Model file for the job. Use its own axes, mm. Round coordinates to 2 decimals unless told otherwise and drop trailing zeros. Loops run counter-clockwise (first coordinate to the right, second up) from the corner with the lowest first, then second, coordinate; pieces in that order, holes last. Notation, with made-up numbers: M 41,30 L 77,30 A23 ccw 77,40 Z; hole C 65,46 d11. An arc over 180 degrees is marked long. Use a Markdown table: item, result. Add a question column.
Q1. Cut at D-D (x = 8). Give the cut face in (y, z), plus the area to 3 significant figures.
Q2. Cut at C-C (x = 18.5). Give the cut face in (y, z).
Q3. Cut at A-A (y = 0). Give the cut face in (x, z).
Q4. Pin check, flat tips, straight feed: pin 1 (10 mm diameter, centred on x = 13.5, z = -24, fed in from -Y); pin 2 (1.5 mm diameter, centred on x = 6.5, y = 10, fed in from -Z); pin 3 (8 mm diameter, centred on x = 15.5, z = 1, fed in from +Y). Stop position of each tip, or through.
Q5. Probe line 1 (Y direction, x = 20.05, z = 0); line 2 (Z direction, x = 3.5, y = -6); line 3 (Y direction, x = 16, z = 4.5). List the from-to ranges inside material, lowest first. Write a range as from..to.
Q6. Mould opens along Z. For faces 1 (the face through (16.626, 21.031, -27.428)), 2 (the face through (11.02, -1.76, -39.96)), 3 (the face through (1, -35, -15)) say: +Z half, -Z half, draft (parallel to the pull), parting line (faces both ways), or undercut.
from build123d import *

# Parameters (mm, degrees)
FILLET1_R = 1.5
FILLET2_R = 0.8
FILLET3_R = 0.4


with BuildPart() as part:
    # Sketch1 → Revolve1 (revolve)
    with BuildSketch(Plane.XY, mode=Mode.PRIVATE) as revolve1_sk:
        Polygon((22, 34.05), (22, 40), (1, 40), (1, 37.317672581), (19.5318921, 34.05), align=None)
    revolve(revolve1_sk.sketch.rotate(Axis((0, 0, 0), (1, 0, 0)), 90), axis=Axis((0, 0, 0), (1, 0, 0)))

    # Fillet1
    fillet1_edges = [part.edges().sort_by_distance(p)[0] for p in [
        (22, 0, -40),
    ]]
    fillet(fillet1_edges, radius=FILLET1_R)

    # Fillet2
    fillet2_edges = [part.edges().sort_by_distance(p)[0] for p in [
        (1, 0, -40),
    ]]
    fillet(fillet2_edges, radius=FILLET2_R)

    # Fillet3
    fillet3_edges = [part.edges().sort_by_distance(p)[0] for p in [
        (22, 0, -34.05),
        (1, 0, -37.317672581),
    ]]
    fillet(fillet3_edges, radius=FILLET3_R)


solid = part.part
Checked values:
| question | item | result |
|---|---|---|
| 1 | outline | C 0,0 d80; hole C 0,0 d72.17 |
| 1 | area | 936 mm^2 |
| 2 | outline | C 0,0 d80; hole C 0,0 d68.46 |
| 3 | outline | M 1,-39.2 A0.8 ccw 1.8,-40 L 20.5,-40 A1.5 ccw 22,-38.5 L 22,-34.45 A0.4 ccw 21.6,-34.05 L 19.53,-34.05 L 1.33,-37.26 A0.4 ccw 1,-37.65 Z; M 1,37.65 A0.4 ccw 1.33,37.26 L 19.53,34.05 L 21.6,34.05 A0.4 ccw 22,34.45 L 22,38.5 A1.5 ccw 20.5,40 L 1.8,40 A0.8 ccw 1,39.2 Z |
| 4 | pin 1 | stops at y = -35.2 |
| 4 | pin 2 | stops at z = -38.92 |
| 4 | pin 3 | stops at y = 40 |
| 5 | line 1 | y = -40..-34.05, 34.05..40 |
| 5 | line 2 | z = -39.55..-36.39, 36.39..39.55 |
| 5 | line 3 | y = -39.75..-34.38, 34.38..39.75 |
| 6 | face 1 | undercut |
| 6 | face 2 | parting line |
| 6 | face 3 | draft |
